Could you check a few things on this model? Use its own coordinates, in mm. A direction names the side the tool comes from. Give positions to 0.01 mm unless a question says otherwise; leave off trailing zeros. Order: outer loops, then holes, each group sorted by start corner. A loop starts at its lowest first (then second) coordinate and runs counter-clockwise, first axis right, second up.
from build123d import *

# Parameters (mm, degrees)
F0_R     = 50.8
F2_R     = 25.4
F5_DEPTH = 60.706


with BuildPart() as f3:
    # F0 (on Front) → F3 section 0
    with BuildSketch(Plane.XZ):
        Circle(F0_R)
    # F2 (on offset) → F3 section 1
    with BuildSketch(Plane.XZ.offset(43.18)):
        Circle(F2_R)
    loft()

    # F4 (on face) → F5 (cut)
    with BuildSketch(Plane.XZ.offset(43.18)):
        Polygon((-3.6808389062, -6.3754), (3.6808389062, -6.3754), (7.3616778124, 0), (3.6808389062, 6.3754), (-3.6808389062, 6.3754), (-7.3616778124, 0), align=None)
    extrude(amount=-F5_DEPTH, mode=Mode.SUBTRACT)


solid = f3.part
Item 1: We'd pull the mould along Z, two halves only. Please class faces 1 (the conical face through (-3.8, -36.3, 29.2)), 2 (the flat face through (5, -43.18, -5)), 3 (the flat face through (-5.55, -21.89, -3.14)): +Z half, -Z half, draft (parallel to the pull), parting line (faces both ways), or undercut.
Findings:
face 1: parting line
face 2: draft
face 3: undercut
Item 2: Imagine slicing it at B-B on y = -27. List the corners of the cut face in (x, z) for me.
Findings:
outline: circle Ø69.84 at (0, 0); hole (-7.36, 0) - (-3.68, -6.38) - (3.68, -6.38) - (7.36, 0) - (3.68, 6.38) - (-3.68, 6.38) - close
Item 3: For faces 4 (the flat face through (11, 0, 1)), 5 (the flat face through (5.495, -21.892, -3.232)), which set-ups out of +Z, -Z, +X, -X, +Y, -Y let a thin tool reach every point of the face, with its end or its side?
Findings:
face 4: +Z, -Z, +X, -X, +Y
face 5: +Y, -Y
Item 4: Imagine slicing it at C-C on y = -17.5. List the corners of the cut face in (x, z) for me.
Findings:
outline: circle Ø81.01 at (0, 0); hole (-7.36, 0) - (-3.68, -6.38) - (3.68, -6.38) - (7.36, 0) - (3.68, 6.38) - (-3.68, 6.38) - close
Item 5: Imagine slicing it at A-A on x = 0. List the corners of the cut face in (y, z) for me.
Findings:
outline: (-43.18, -25.4) - (0, -50.8) - (0, -6.38) - (-43.18, -6.38) - close; (-43.18, 6.38) - (0, 6.38) - (0, 50.8) - (-43.18, 25.4) - close
Item 6: Please list where these lines run through material, in increasing order: line 1 along X through (y, z) = (-5.5, -3); line 2 along Z through (x, y) = (-8, -30); line 3 along Y through (x, z) = (39.5, 29).
Findings:
line 1: x = -47.47 to -5.63, 5.63 to 47.47
line 2: z = -32.17 to 32.17
line 3: y = -3.06 to 0
Item 7: For pin 1 (10 mm diameter, centred on y = -11.5, z = -3.5, fed in from -X); pin 2 (2 mm diameter, centred on y = -17.5, z = 23.5, fed in from -X); pin 3 (6 mm diameter, centred on y = -22.5, z = -13, fed in from +X), each with a flat end and sliding along its axis, tell me the tip position at first contact or that it passes through.
Findings:
pin 1: stops at x = -46.87
pin 2: stops at x = -33.99
pin 3: stops at x = 37.37
